For this review, take the finished solid that the model builds, in its own axes (mm). Face numbers are marked on the shaded views. Give positions to 0.01 mm unless a question says otherwise; leave off trailing zeros. Write each loop counter-clockwise with the first axis right and the second up, starting at its lowest first coordinate (ties: lowest second). Pieces come first, ordered by that corner, then holes. Notation, with made-up numbers: M 2,37 L 26,37 A8 ccw 26,48 Z; hole C -1.5,-36 d11. An arc over 180 degrees is marked long. Use one line per item in the form item = value. Start each with the question number.
Q1. Consider section B-B on x = 0. Write out the cut boundary in (y, z), and give its area (3 significant figures).
Q2. Mouldability with a two-part tool opening along X and no side actions: class the marked faces 1, 2 and 3 as released by +X, released by -X, zero draft, split by the parting line, or undercut.
Q3. For probe 1 along Y at (x, z) = (56, 101.5); probe 2 along Y at (x, z) = (40, -92); probe 3 along Z at (x, y) = (0, -159.3), list the stretches that pass through material, from the lowest coordinate up. Write a range as [from, to].
Q4. Consider section C-C on y = -118. Write out the cut boundary in (x, z).
Q5. Consider section A-A on z = 95.5. Write out the cut boundary in (x, y).
Q6. Clearance check with flat-ended pins moving along their axes: pin 1 Ø6 at (x, y) = (-6.5, -125.5) entering from +Z; pin 2 Ø12.5 at (x, z) = (-45.5, 135) entering from +Y; pin 3 Ø4 at (x, z) = (-7.5, -41.5) entering from -Y. State where each tip first meets the part, or that it passes through.
Q7. Consider section D-D on y = -20. Write out the cut boundary in (x, z).
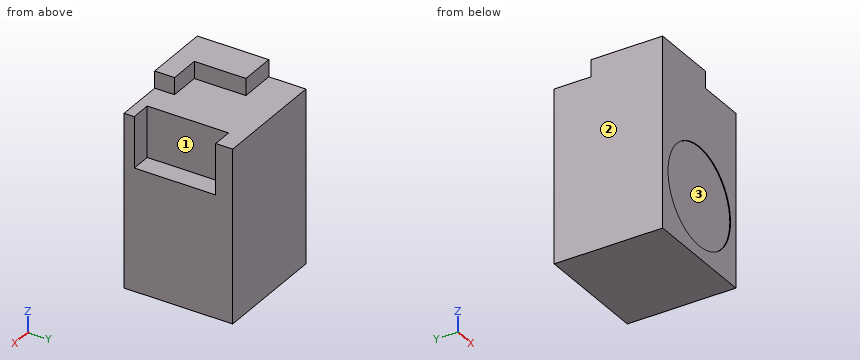
```python
from build123d import *

# Parameters (mm, degrees)
F0_W     = 170
F0_H     = 255
F1_DEPTH = 160
F2_R     = 72.5
F3_DEPTH = 1
F4_W     = 120
F4_H     = 75
F5_DEPTH = 30
F7_DEPTH = 25


with BuildPart() as f1:
    # F0 (on Front) → F1 (new body)
    with BuildSketch(Plane.XZ):
        Rectangle(F0_W, F0_H)
    extrude(amount=F1_DEPTH)

    # F2 (on face) → F3 (cut)
    with BuildSketch(Plane.XZ.offset(160)):
        with Locations((0, -37.5)):
            Circle(F2_R)
    extrude(amount=-F3_DEPTH, mode=Mode.SUBTRACT)

    # F4 (on face) → F5 (cut)
    with BuildSketch(Plane.YZ.offset(85)):
        with Locations((-85, 90)):
            Rectangle(F4_W, F4_H)
    extrude(amount=-F5_DEPTH, mode=Mode.SUBTRACT)

    # F6 (on face) → F7 (join)
    with BuildSketch(Plane.XY.offset(127.5)):
        Polygon((-85, -130.726978), (-85, -160), (13.915417, -160), (13.915417, -130.726978), (-31.836193, -130.726978), (-31.836193, -54.676291), (-85, -54.676291), align=None)
    extrude(amount=F7_DEPTH)


solid = f1.part
```
Working result:
q1.outline = M -160,-127.5 L 0,-127.5 L 0,127.5 L -130.73,127.5 L -130.73,152.5 L -160,152.5 L -160,35 L -159,35 L -159,-110 L -160,-110 Z
q1.area = 41,400 mm²
q2.face_1 = released by +X
q2.face_2 = released by -X
q2.face_3 = undercut
q3.probe_1 = [-160, -145], [-25, 0]
q3.probe_2 = [-159, 0]
q3.probe_3 = [-127.5, -110], [35, 152.5]
q4.outline = M -85,-127.5 L 85,-127.5 L 85,52.5 L 55,52.5 L 55,127.5 L -31.84,127.5 L -31.84,152.5 L -85,152.5 Z
q5.outline = M -85,-160 L 85,-160 L 85,-145 L 55,-145 L 55,-25 L 85,-25 L 85,0 L -85,0 Z
q6.pin_1 = 127.5
q6.pin_2 = -54.68
q6.pin_3 = -159
q7.outline = M -85,-127.5 L 85,-127.5 L 85,127.5 L -85,127.5 Z
